from build123d import *

# Parameters (mm, degrees)
F0_R      = 14
F1_DEPTH  = 2
F3_DEPTH  = 25
F4_R      = 10.6
F5_DEPTH  = 5
F7_R      = 14
F8_DEPTH  = 23.5
F9_W      = 10
F9_H      = 3
F10_DEPTH = 27
F11_DEPTH = 5


with BuildPart() as f1:
    # F0 (on Right) → F1 (new body)
    with BuildSketch(Plane.YZ):
        with BuildLine():
            Line((-17.5, 0), (-17.5, -17))
            Line((-17.5, -17), (0, -17))
            Line((0, -17), (17.5, -17))
            Line((17.5, -17), (17.5, 0))
            Line((17.5, 0), (14.628571, 6.481119))
            ThreePointArc((14.628571, 6.481119), (0, 16), (-14.628571, 6.481119))
            Line((-14.628571, 6.481119), (-17.5, 0))
        make_face()
        Circle(F0_R, mode=Mode.SUBTRACT)
    extrude(amount=F1_DEPTH)

    # F2 (on face) → F3 (join)
    with BuildSketch(Plane.YZ.offset(2)):
        Polygon((-11.934718, -1.25), (-11.934718, 1.25), (-16.946193, 1.25), (-17.5, 0), (-17.5, -17), (-13.944085, -17), (-13.944085, -1.25), align=None)
        Polygon((11.934718, 1.25), (11.934718, -1.25), (13.944085, -1.25), (13.944085, -17), (17.5, -17), (17.5, 0), (16.946193, 1.25), align=None)
    extrude(amount=F3_DEPTH)

    # F4 (on Right) → F5 (join)
    with BuildSketch(Plane.YZ):
        with BuildLine():
            Line((0, -17), (17.5, -17))
            Line((17.5, -17), (17.5, 0))
            Line((17.5, 0), (14.628571, 6.481119))
            ThreePointArc((14.628571, 6.481119), (0, 16), (-14.628571, 6.481119))
            Line((-14.628571, 6.481119), (-17.5, 0))
            Line((-17.5, 0), (-17.5, -17))
            Line((-17.5, -17), (0, -17))
        make_face()
        Circle(F4_R, mode=Mode.SUBTRACT)
    extrude(amount=-F5_DEPTH)

    # F7 (on offset) → F8 (cut)
    with BuildSketch(Plane.YZ.offset(23.5)):
        Circle(F7_R)
    extrude(amount=-F8_DEPTH, mode=Mode.SUBTRACT)

    # F9 (on Right) → F10 (join)
    with BuildSketch(Plane.YZ):
        with Locations((-8.944085, -15.5)):
            Rectangle(F9_W, F9_H)
        with Locations((8.944085, -15.5)):
            Rectangle(F9_W, F9_H)
    extrude(amount=F10_DEPTH)

    # F9 (on Right) → F11 (join)
    with BuildSketch(Plane.YZ):
        with Locations((-8.944085, -15.5)):
            Rectangle(F9_W, F9_H)
        with Locations((8.944085, -15.5)):
            Rectangle(F9_W, F9_H)
    extrude(amount=-F11_DEPTH)


solid = f1.part
Check sheet for the modelled part. Datum: model origin and axes. Units: mm. A direction names the side the tool comes from. Round coordinates to 2 decimals unless told otherwise and drop trailing zeros. Loops run counter-clockwise (first coordinate to the right, second up) from the corner with the lowest first, then second, coordinate; pieces in that order, holes last. Notation, with made-up numbers: (-8.5, -23.5) -> (25.5, -23.5) arc R29 ccw to (25.5, 3.5) -> close; hole circle Ø10 at (51, -6.5). An arc over 180 degrees is marked (long way). Put each result on its own line as item: value. Start each with the question number.
1. Gauge pin test, flat ends, axial feed: pin 1 (1 mm diameter, centred on x = 16.5, y = 4, fed in from +Z); pin 2 (4.5 mm diameter, centred on y = -5, z = -12, fed in from +X); pin 3 (8 mm diameter, centred on x = 19, y = -12.5, fed in from +Z); pin 4 (2 mm diameter, centred on x = 11.5, z = 2.5, fed in from +Y) (3 decimals). Record the tip position at first contact, or that the pin passes through.
2. Access from +Z, -Z, +X, -X, +Y, -Y to the whole of each face (thin tool, end or side, straight path). Record for faces 4 (the face through (5, -14, 0)), 5 (the face through (14, -16, 1.25)), 6 (the face through (25, -11.935, 0)), 7 (the face through (25, 13, -1.25)), 8 (the face through (-1.451, -16.044, 3.286)).
3. Scan lines: probe 1 along Z at (x, y) = (-2.2, 0); probe 2 along Y at (x, z) = (16, -13); probe 3 along Z at (x, y) = (24, -12). Record each from-to range of solid material in increasing order.
4. Section check D-D (y = -7). Enter the section's corners in (x, z), plus the area to 3 significant figures.
5. Section check A-A (y = 0). Enter the section's corners in (x, z).
6. Section check C-C (z = -3.5). Enter the section's corners in (x, y), plus the area to 3 significant figures.
7. Section check B-B (x = 22). Enter the section's corners in (y, z).
8. Draft check along X on faces 1 (the face through (2, 0, 15)), 2 (the face through (23.5, 13, 0)), 3 (the face through (25, -13, -1.25)). Enter one of: +X half, -X half, draft (parallel to the pull), parting line (faces both ways), or undercut.
Findings:
1. pin 1: stops at z = -14
1. pin 2: stops at x = 27
1. pin 3: stops at z = 1.25
1. pin 4: passes through
2. face 4: none
2. face 5: +Z, +X, +Y, -Y
2. face 6: +Z, +X
2. face 7: +X
2. face 8: +Z, +X, -X, -Y
3. probe 1: z = -17 to -10.6, 10.6 to 16
3. probe 2: y = -17.5 to -13.94, 13.94 to 17.5
3. probe 3: z = -17 to -14, -1.25 to 1.25
4. outline: (-5, -17) -> (27, -17) -> (27, -14) -> (2, -14) -> (2, -12.12) -> (0, -12.12) -> (0, -7.96) -> (-5, -7.96) -> close; (-5, 7.96) -> (0, 7.96) -> (0, 12.12) -> (2, 12.12) -> (2, 14.39) -> (-5, 14.39) -> close
4. area: 167 mm^2
5. outline: (-5, -17) -> (2, -17) -> (2, -14) -> (0, -14) -> (0, -10.6) -> (-5, -10.6) -> close; (-5, 10.6) -> (0, 10.6) -> (0, 14) -> (2, 14) -> (2, 16) -> (-5, 16) -> close
6. outline: (-5, -17.5) -> (27, -17.5) -> (27, -13.94) -> (2, -13.94) -> (2, -13.56) -> (0, -13.56) -> (0, -10.01) -> (-5, -10.01) -> close; (-5, 10.01) -> (0, 10.01) -> (0, 13.56) -> (2, 13.56) -> (2, 13.94) -> (27, 13.94) -> (27, 17.5) -> (-5, 17.5) -> close
6. area: 269 mm^2
7. outline: (-17.5, -17) -> (-3.94, -17) -> (-3.94, -14) -> (-13.94, -14) -> (-13.94, -1.25) arc R14 cw to (-13.94, 1.25) -> (-16.95, 1.25) -> (-17.5, 0) -> close; (3.94, -17) -> (17.5, -17) -> (17.5, 0) -> (16.95, 1.25) -> (13.94, 1.25) arc R14 cw to (13.94, -1.25) -> (13.94, -14) -> (3.94, -14) -> close
8. face 1: +X half
8. face 2: undercut
8. face 3: draft
